from build123d import *

# Parameters (mm, degrees)
SKETCH1_R                   = 10.2489
BOSS_EXTRUDE1_DEPTH         = 2.9845
BOSS_EXTRUDE1_2_DEPTH       = 2.9845
SKETCH2_R                   = 10.2489
BOSS_EXTRUDE2_DEPTH         = 5.08
BOSS_EXTRUDE3_DEPTH         = 3.81
F_1_4_0_25_DIAMETER_HOLE1_D = 6.35
BOSS_EXTRUDE4_DEPTH         = 17.78
SKETCH8_R                   = 2.25
CUT_EXTRUDE1_DEPTH          = 17.78
SKETCH9_W                   = 17.78
SKETCH9_H                   = 2.54
BOSS_EXTRUDE5_DEPTH         = 17.78
CUT_EXTRUDE2_REACH          = 251.039
CUT_EXTRUDE3_DEPTH          = 20
BOSS_EXTRUDE6_DEPTH         = 2.54
BOSS_EXTRUDE7_DEPTH         = 39.624
CUT_EXTRUDE5_DEPTH          = 6.35
F_6_CLEARANCE_HOLE1_D       = 3.7973
SKETCH19_W                  = 39.624
SKETCH19_H                  = 13.560471889
BOSS_EXTRUDE8_DEPTH         = 6.35
M4_CLEARANCE_HOLE1_D        = 4.5
SKETCH20_R                  = 4.308
CUT_EXTRUDE6_DEPTH          = 195.822050963
FILLET1_R                   = 11
CUT_EXTRUDE7_DEPTH          = 6.35
BOSS_EXTRUDE9_DEPTH         = 21.844


with BuildPart() as part:
    # Sketch1 → Boss-Extrude1 (new body)
    with BuildSketch(Plane.XY):
        Circle(SKETCH1_R)
    extrude(amount=BOSS_EXTRUDE1_DEPTH)



with BuildPart() as body_2:
    # Sketch1 → Boss-Extrude1 2 (new body)
    with BuildSketch(Plane.XY):
        with Locations((-72.411066703, 81.765798589)):
            Circle(SKETCH1_R)
    extrude(amount=BOSS_EXTRUDE1_2_DEPTH)


with BuildPart() as part_1:
    add(part.part)

    add(body_2.part)  # Boss-Extrude2 merges body 2
    # Sketch2 → Boss-Extrude2 (add)
    with BuildSketch(Plane.XY.offset(2.9845)):
        with Locations((-72.411066703, 81.765798589)):
            Circle(SKETCH2_R)
        Circle(SKETCH2_R)
    extrude(amount=BOSS_EXTRUDE2_DEPTH)

    # Sketch3 → Boss-Extrude3 (add)
    with BuildSketch(Plane.XY.offset(8.0645)):
        Polygon((-134.069705847, 103.500499391), (-96.039101852, 137.180065299), (52.150988145, -30.154592279), (14.12038415, -63.834158187), align=None)
    extrude(amount=BOSS_EXTRUDE3_DEPTH)

    # 1/4 (0.25) Diameter Hole1 (through all)
    with Locations(Plane.XY.offset(11.8745)):
        with Locations((0, 0), (-72.411066703, 81.765798589)):
            Hole(F_1_4_0_25_DIAMETER_HOLE1_D / 2)

    # Sketch7 → Boss-Extrude4 (add)
    with BuildSketch(Plane(origin=(0, 0, 8.0645), x_dir=(-1, 0, 0), z_dir=(0, 0, -1))):
        Polygon((53.34482504, 12.346831233), (66.604496657, 27.319509971), (61.850671158, 31.529455709), (48.59099954, 16.556776971), align=None)
        Polygon((120.810034229, 88.527820652), (134.069705847, 103.500499391), (129.315880348, 107.710445129), (116.05620873, 92.737766391), align=None)
    extrude(amount=BOSS_EXTRUDE4_DEPTH)

    # Sketch8 → Cut-Extrude1 (cut)
    with BuildSketch(Plane(origin=(-19.015301997, -16.839782954, 0), x_dir=(0, 0, -1), z_dir=(0.7486339369082552, 0.6629835808745542, 0))):
        with Locations(Location((0.8255, 54.61, 0), (0, 0, 90))):
            Circle(SKETCH8_R)
        with Locations(Location((0.8255, 156.37, 0), (0, 0, 90))):
            Circle(SKETCH8_R)
    extrude(amount=-CUT_EXTRUDE1_DEPTH, mode=Mode.SUBTRACT)

    # Sketch9 → Boss-Extrude5 (add)
    with BuildSketch(Plane(origin=(-19.015301997, -16.839782954, 0), x_dir=(0, 0, -1), z_dir=(0.7486339369082552, 0.6629835808745542, 0))):
        with Locations((0.8255, 63.34)):
            Rectangle(SKETCH9_W, SKETCH9_H)
        with Locations((0.8255, 45.88)):
            Rectangle(SKETCH9_W, SKETCH9_H)
        with Locations((0.8255, 165.1)):
            Rectangle(SKETCH9_W, SKETCH9_H)
        with Locations((0.8255, 147.64)):
            Rectangle(SKETCH9_W, SKETCH9_H)
    extrude(amount=BOSS_EXTRUDE5_DEPTH)

    # Cut-Extrude2: up to this face of the body (flat: up to its plane)
    cut_extrude2_end = Plane(part_1.part.faces().sort_by_distance((-111.777765781, 96.526717556, -0.8255))[0])
    # Sketch10 → Cut-Extrude2 (cut, up to the picked face)
    with BuildSketch(Plane(origin=(-110.30057835, 124.550228083, 0), x_dir=(0.7486339369082557, 0.6629835808745536, 0), z_dir=(-0.6629835808745536, 0.7486339369082557, 0)), mode=Mode.PRIVATE) as cut_extrude2_sk1:
        Polygon((-7.62, 9.7155), (-7.62, -8.0645), (-25.4, 9.7155), align=None)
    cut_extrude2_tool1 = split(extrude(cut_extrude2_sk1.sketch, amount=-CUT_EXTRUDE2_REACH, mode=Mode.PRIVATE), bisect_by=cut_extrude2_end, keep=Keep.BOTH, mode=Mode.PRIVATE)
    add(cut_extrude2_tool1.solids().sort_by(Axis((-120.442073, 115.569011, -3.788833), (0.6629835808745536, -0.7486339369082557, 0)))[0], mode=Mode.SUBTRACT)

    # Sketch11 → Cut-Extrude3 (cut)
    with BuildSketch(Plane(origin=(-42.83536916, 48.369238664, 0), x_dir=(0.7486339369082559, 0.6629835808745536, 0), z_dir=(-0.6629835808745536, 0.7486339369082559, 0))):
        Polygon((-7.62, 9.7155), (-7.62, -8.0645), (-25.4, 9.7155), align=None)
    extrude(amount=-CUT_EXTRUDE3_DEPTH, mode=Mode.SUBTRACT)

    # Sketch13 → Boss-Extrude6 (add)
    with BuildSketch(Plane(origin=(-110.30057835, 124.550228083, 0), x_dir=(0.7486339369082557, 0.6629835808745536, 0), z_dir=(-0.6629835808745536, 0.7486339369082557, 0))):
        Polygon((-25.4, 9.7155), (19.05, 9.7155), (19.05, -8.0645), (-7.62, -8.0645), align=None)
    extrude(amount=-BOSS_EXTRUDE6_DEPTH)

    # Sketch14 → Boss-Extrude7 (add)
    with BuildSketch(Plane(origin=(0, 0, 8.0645), x_dir=(-1, 0, 0), z_dir=(0, 0, -1))):
        Polygon((-52.150988145, -30.154592279), (-14.12038415, -63.834158187), (-5.700492673, -54.326507188), (-43.731096668, -20.64694128), align=None)
    extrude(amount=BOSS_EXTRUDE7_DEPTH)

    # Sketch15 → Cut-Extrude5 (cut)
    with BuildSketch(Plane.XY.offset(11.8745)):
        Polygon((38.433391408, -33.820658256), (42.550325055, -30.174738298), (37.334398928, -28.432329153), (33.21746528, -32.078249111), (33.824088825, -35.052507224), align=None)
        Polygon((43.649317536, -35.563067402), (43.042693991, -32.588809289), (38.433391408, -33.820658256), (34.31645776, -37.466578215), (39.532383888, -39.20898736), align=None)
        Polygon((38.433391408, -33.820658256), (43.042693991, -32.588809289), (42.550325055, -30.174738298), align=None)
        Polygon((34.31645776, -37.466578215), (38.433391408, -33.820658256), (33.824088825, -35.052507224), align=None)
        Polygon((21.198191786, -46.233889763), (19.41808941, -50.660441211), (23.535023058, -47.014521252), align=None)
        Polygon((15.301155763, -54.306361169), (17.637987035, -55.086992658), (19.41808941, -50.660441211), align=None)
        Polygon((14.202163283, -48.918032065), (15.301155763, -54.306361169), (19.41808941, -50.660441211), (21.198191786, -46.233889763), (18.31909693, -45.272112107), align=None)
        Polygon((19.41808941, -50.660441211), (17.637987035, -55.086992658), (20.51708189, -56.048770314), (24.634015538, -52.402850356), (23.535023058, -47.014521252), align=None)
    extrude(amount=-CUT_EXTRUDE5_DEPTH, mode=Mode.SUBTRACT)

    # #6 Clearance Hole1 (through all)
    with Locations(Plane.XY.offset(5.5245)):
        with Locations((19.41808941, -50.660441211), (38.433391408, -33.820658256)):
            Hole(F_6_CLEARANCE_HOLE1_D / 2)

    # Sketch19 → Boss-Extrude8 (add)
    with BuildSketch(Plane(origin=(-23.769127497, -21.049728693, 0), x_dir=(0, 0, 1), z_dir=(-0.7486339369082559, -0.6629835808745536, 0))):
        with Locations((-11.7475, -37.669764056)):
            Rectangle(SKETCH19_W, SKETCH19_H)
    extrude(amount=-BOSS_EXTRUDE8_DEPTH)

    # M4 Clearance Hole1 (through all)
    with Locations(Plane(origin=(-19.015301997, -16.839782954, 0), x_dir=(0, 0, -1), z_dir=(0.7486339369082555, 0.6629835808745539, 0))):
        with Locations((1.866346616, -40.889528111), (21.728039849, -40.889528111)):
            Hole(M4_CLEARANCE_HOLE1_D / 2)

    # Sketch20 → Cut-Extrude6 (cut, through all)
    with BuildSketch(Plane(origin=(-19.015301997, -16.839782954, 0), x_dir=(0, 0, -1), z_dir=(0.7486339369082555, 0.6629835808745539, 0))):
        with Locations((21.728039849, -40.889528111)):
            Circle(SKETCH20_R)
        with Locations((1.866346616, -40.889528111)):
            Circle(SKETCH20_R)
    extrude(amount=CUT_EXTRUDE6_DEPTH, mode=Mode.SUBTRACT)

    # Fillet1
    # the kernel refuses this fillet: 11 mm, written as the material it adds along each edge
    with BuildSketch(Plane(origin=(-127.631902052, 105.808914929, 8.0645), x_dir=(0.6629835808745532, -0.7486339369082561, 1.2918958832001814e-15), z_dir=(0.7486339369082562, 0.6629835808745532, 0))) as fillet1_piece_1:
        with BuildLine():
            CenterArc((FILLET1_R, FILLET1_R), FILLET1_R, 180, 90)
            Line((0, FILLET1_R), (0, 0))
            Line((0, 0), (FILLET1_R, 0))
        make_face()
    extrude(amount=44.45)
    # the kernel refuses this fillet: 11 mm, written as the material it takes off along each edge
    with BuildSketch(Plane(origin=(-154.657139112, 85.268450917, 11.8745), x_dir=(0, 0, -1), z_dir=(0.7486339369082557, 0.6629835808745537, 0))) as fillet1_2_piece_1:
        with BuildLine():
            CenterArc((FILLET1_R, -FILLET1_R), FILLET1_R, 90, 90)
            Line((0, -FILLET1_R), (0, 0))
            Line((0, 0), (FILLET1_R, 0))
        make_face()
    extrude(amount=105.8, mode=Mode.SUBTRACT)
    with BuildSketch(Plane(origin=(72.73842141, -11.922543805, 11.8745), x_dir=(-0.6629835808745536, 0.7486339369082557, 0), z_dir=(-0.7486339369082559, -0.6629835808745537, 0))) as fillet1_2_piece_2:
        with BuildLine():
            CenterArc((FILLET1_R, FILLET1_R), FILLET1_R, 180, 90)
            Line((0, FILLET1_R), (0, 0))
            Line((0, 0), (FILLET1_R, 0))
        make_face()
    extrude(amount=105.8, mode=Mode.SUBTRACT)

    # Sketch23 → Cut-Extrude7 (cut)
    with BuildSketch(Plane.XY.offset(5.5245)):
        Polygon((37.334398928, -28.432329153), (33.21746528, -32.078249111), (34.31645776, -37.466578215), (39.532383888, -39.20898736), (43.649317536, -35.563067402), (42.550325055, -30.174738298), align=None)
        Polygon((14.202163283, -48.918032065), (15.301155763, -54.306361169), (20.51708189, -56.048770314), (24.634015538, -52.402850356), (23.535023058, -47.014521252), (18.31909693, -45.272112107), align=None)
    extrude(amount=-CUT_EXTRUDE7_DEPTH, mode=Mode.SUBTRACT)

    # Sketch24 → Boss-Extrude9 (add)
    with BuildSketch(Plane(origin=(0, 0, -9.7155), x_dir=(-1, 0, 0), z_dir=(0, 0, -1))):
        Polygon((117.740187025, 94.639296591), (116.05620873, 92.737766391), (120.810034229, 88.527820652), (134.069705847, 103.500499391), (96.039101852, 137.180065299), (94.355123557, 135.278535099), (127.631902052, 105.808914929), align=None)
    extrude(amount=BOSS_EXTRUDE9_DEPTH)


solid = part_1.part
Can you work these out from the model? Positions are in its coordinate system, mm. A direction names the side the tool comes from. Coordinates: 2 decimals unless noted, no trailing zeros. Write each loop counter-clockwise with the first axis right and the second up, starting at its lowest first coordinate (ties: lowest second). Pieces come first, ordered by that corner, then holes. Notation, with made-up numbers: (33.25, -14) - (87.25, -14) arc R13 ccw to (87.25, -5) - close; hole circle Ø5 at (34, 82). An arc over 180 degrees is marked (long way). Return JSON: item names as keys, results as strings. Group by question number.
Item 1: I'm going to push flat-ended pins straight in: pin 1 Ø5 at (x, z) = (5, -4.5) entering from -Y; pin 2 Ø9 at (x, y) = (-58.5, 22.5) entering from -Z; pin 3 Ø2 at (x, z) = (21, -12.5) entering from -Y; pin 4 Ø5 at (x, y) = (38.43, -33.82) entering from -Z. Where does each tip first touch, or does it pass through?
Item 2: If we section it at B-B (y = 0): Write out the boundary of the cut face in (x, z) (1 decimal).
Item 3: We'd pull the mould along X, two halves only. Please class faces 1 (the face through (31.32, -44.41, 8.57)), 2 (the face through (41, -34, -0.825)), 3 (the face through (-75, 84, 0)): pulls with the +X half, pulls with the -X half, needs draft (parallel to the pull), parting line crosses it, or undercut.
Item 4: If we section it at C-C (y = 57.5): Write out the boundary of the cut face in (x, z).
Item 5: Please list where these lines run through material, in increasing order: probe 1 along Y at (x, z) = (0, 2.5) (3 decimals); probe 2 along Z at (x, y) = (2.5, -19); probe 3 along Y at (x, z) = (18, -19).
Item 6: Which directions (+Z, -Z, +X, -X, +Y, -Y) give clear straight access to the entire face, cutting with the end or side of a thin tool? Please do faces 4 (the face through (-110.16, 99.68, -0.7)), 5 (the face through (-0.95, -42.1, -12.02)), 6 (the face through (27.355, -36.148, -21.692)), 7 (the face through (26.86, -35.59, -27.8)).
Item 7: If we section it at A-A (x = -73): Write out the boundary of the cut face in (y, z), then the cut area to 3 significant figures.
Return value:
{
 "1": {"pin 1": "stops at y = -56.36", "pin 2": "stops at z = -9.72", "pin 3": "stops at y = -58.63", "pin 4": "stops at z = -31.56"},
 "2": {"outline": "(-42.4, 8.1) - (-10.2, 8.1) - (-10.2, 0) - (-3.2, 0) - (-3.2, 11.9) - (-42.4, 11.9) - close; (3.2, 0) - (10.2, 0) - (10.2, 8.1) - (25.4, 8.1) - (25.4, 11.9) - (3.2, 11.9) - close"},
 "3": {"face 1": "pulls with the +X half", "face 2": "undercut", "face 3": "needs draft"},
 "4": {"outline": "(-93.33, 8.06) - (-25.48, 8.06) - (-25.48, 11.87) - (-93.33, 11.87) - close"},
 "5": {"probe 1": "y = -47.89 to -41.261, -10.249 to -3.175, 3.175 to 10.249", "probe 2": "z = 8.06 to 11.87", "probe 3": "y = -60.4 to -51.92, -49.4 to -43.43"},
 "6": {"face 4": "-Z, +X", "face 5": "-Z, -X", "face 6": "+Y", "face 7": "-Z, +Y"},
 "7": {"outline": "(34.54, 8.06) - (71.53, 8.06) - (71.53, 0) - (78.65, 0) - (78.65, 11.87) - (34.54, 11.87) - close; (84.89, 0) - (92, 0) - (92, 8.06) - (111.16, 8.06) - (111.16, 11.87) - (84.89, 11.87) - close", "area": "383 mm^2"}
}
